from build123d import *

# Parameters (mm, degrees)
SKETCH1_W                 = 8.5
SKETCH1_H                 = 60.8
BOSS_EXTRUDE1_DEPTH       = 4.75
F_3_0MM_DOWEL_HOLE1_D     = 3
F_3_0MM_DOWEL_HOLE1_DEPTH = 5
F_3_0MM_DOWEL_HOLE1_TIP   = 0.901290929
SKETCH6_R                 = 2.85
CUT_EXTRUDE1_DEPTH        = 2.2


with BuildPart() as part:
    # Sketch1 → Boss-Extrude1 (new body)
    with BuildSketch(Plane.XY):
        with Locations((4.25, -30.4)):
            Rectangle(SKETCH1_W, SKETCH1_H)
    extrude(amount=BOSS_EXTRUDE1_DEPTH)

    # Ø3.0mm Dowel Hole1
    with Locations(Plane.XY.offset(4.75)):
        with Locations((4.25, -18.2), (4.25, -45.6)):
            Hole(F_3_0MM_DOWEL_HOLE1_D / 2, depth=F_3_0MM_DOWEL_HOLE1_DEPTH)
            with Locations((0, 0, -(F_3_0MM_DOWEL_HOLE1_DEPTH + F_3_0MM_DOWEL_HOLE1_TIP / 2))):  # 118° drill point
                Cone(0, F_3_0MM_DOWEL_HOLE1_D / 2, F_3_0MM_DOWEL_HOLE1_TIP, mode=Mode.SUBTRACT)

    # Sketch6 → Cut-Extrude1 (cut)
    with BuildSketch(Plane.XY.offset(4.75)):
        with Locations((4.25, -18.2)):
            Circle(SKETCH6_R)
        with Locations((4.25, -45.6)):
            Circle(SKETCH6_R)
    extrude(amount=-CUT_EXTRUDE1_DEPTH, mode=Mode.SUBTRACT)


solid = part.part
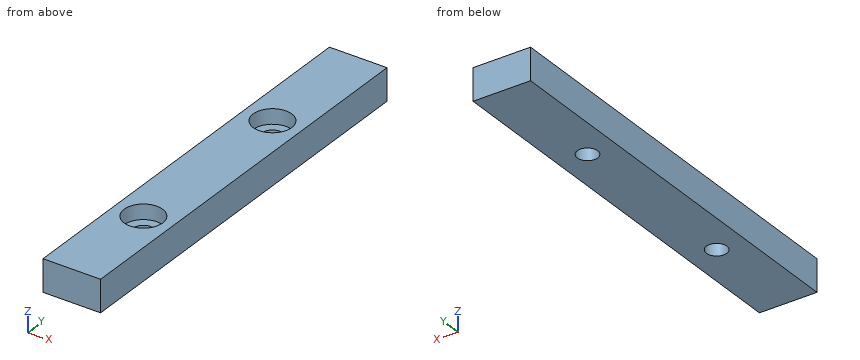
Design review of the part built by this model. Coordinates are the model's own, in mm. Coordinates: 2 decimals unless noted, no trailing zeros. Order: outer loops, then holes, each group sorted by start corner. A loop starts at its lowest first (then second) coordinate and runs counter-clockwise, first axis right, second up.
Item 1: For pin 1 Ø1.8 at (x, y) = (4.25, -18.2) entering from +Z; pin 2 Ø5 at (x, y) = (4.25, -45.6) entering from +Z, all flat-tipped, find the tip position at first contact; note any pin that passes through.
Item 2: Take a section at B-B, the plane z = 1.95. Write out the cut boundary in (x, y).
Item 3: Take a section at A-A, the plane y = -18.2. Write out the cut boundary in (x, z), then the cut area to 3 significant figures.
Item 4: Take a section at C-C, the plane x = 6.5. Write out the cut boundary in (y, z).
Item 5: For line 1 (Y direction, x = 4.25, z = 3.35); line 2 (Y direction, x = 4.25, z = 1.45); line 3 (X direction, y = -20, z = 4.4), list the stretches that pass through material, from the lowest coordinate up.
The answers:
1. pin 1: passes through
1. pin 2: stops at z = 2.55
2. outline: (0, -60.8) - (8.5, -60.8) - (8.5, 0) - (0, 0) - close; hole circle Ø3 at (4.25, -45.6); hole circle Ø3 at (4.25, -18.2)
3. outline: (0, 0) - (2.75, 0) - (2.75, 2.55) - (1.4, 2.55) - (1.4, 4.75) - (0, 4.75) - close; (5.75, 0) - (8.5, 0) - (8.5, 4.75) - (7.1, 4.75) - (7.1, 2.55) - (5.75, 2.55) - close
3. area: 20.2 mm2
4. outline: (-60.8, 0) - (0, 0) - (0, 4.75) - (-16.45, 4.75) - (-16.45, 2.55) - (-19.95, 2.55) - (-19.95, 4.75) - (-43.85, 4.75) - (-43.85, 2.55) - (-47.35, 2.55) - (-47.35, 4.75) - (-60.8, 4.75) - close
5. line 1: y = -60.8 to -48.45, -42.75 to -21.05, -15.35 to 0
5. line 2: y = -60.8 to -47.1, -44.1 to -19.7, -16.7 to 0
5. line 3: x = 0 to 2.04, 6.46 to 8.5
